Check sheet for the modelled part. Datum: model origin and axes. Units: mm. A direction names the side the tool comes from. Give positions to 0.01 mm unless a question says otherwise; leave off trailing zeros. Write each loop counter-clockwise with the first axis right and the second up, starting at its lowest first coordinate (ties: lowest second). Pieces come first, ordered by that corner, then holes. Notation, with made-up numbers: (-19, 36.25) - (-8, 36.25) arc R17 cw to (-8, 56.25) - close; hole circle Ø9 at (-36.75, 8.5). An arc over 180 degrees is marked (long way). Return JSON: item names as keys, results as strings. Group by question number.
```python
from build123d import *

# Parameters (mm, degrees)
F0_W     = 43.2
F0_H     = 4
F1_DEPTH = 1
F0_W_2   = 15.8
F0_H_2   = 2
F0_H_3   = 8.5
F2_DEPTH = 2.5
F3_DEPTH = 5
F4_DEPTH = 8


with BuildPart() as f1:
    # F0 (on Top) → F1 (new body)
    with BuildSketch(Plane.XY):
        Polygon((59, 16.5), (59, 24.5), (43.2, 24.5), (43.2, 20.5), (43.2, 16.5), align=None)
        with Locations((21.6, 22.5)):
            Rectangle(F0_W, F0_H)
    extrude(amount=F1_DEPTH)



with BuildPart() as f1b:
    # F0 (on Top) → F1, piece 2 (new body)
    with BuildSketch(Plane.XY):
        Polygon((59, 0), (59, 8), (43.2, 8), (43.2, 4), (43.2, 0), align=None)
        with Locations((21.6, 2)):
            Rectangle(F0_W, F0_H)
    extrude(amount=F1_DEPTH)


with BuildPart() as f1_1:
    add(f1.part)

    add(f1b.part)  # F2 merges F1b
    # F0 (on Top) → F2 (join)
    with BuildSketch(Plane.XY):
        with Locations((51.1, 25.5)):
            Rectangle(F0_W_2, F0_H_2)
        with Locations((51.1, 12.25)):
            Rectangle(F0_W_2, F0_H_3)
        with Locations((51.1, -1)):
            Rectangle(F0_W_2, F0_H_2)
        Polygon((61, 26.5), (59, 26.5), (59, 24.5), (59, 16.5), (59, 8), (59, 0), (59, -2), (61, -2), align=None)
    extrude(amount=F2_DEPTH)

    # F0 (on Top) → F3 (join)
    with BuildSketch(Plane.XY):
        Polygon((43.2, 8), (43.2, 16.5), (43.2, 20.5), (0, 20.5), (0, 4), (43.2, 4), align=None)
    extrude(amount=F3_DEPTH)

    # F0 (on Top) → F4 (join)
    with BuildSketch(Plane.XY):
        Polygon((43.2, 24.5), (43.2, 26.5), (-2, 26.5), (-2, -2), (43.2, -2), (43.2, 0), (0, 0), (0, 4), (0, 20.5), (0, 24.5), align=None)
    extrude(amount=F4_DEPTH)


solid = f1_1.part
```
Item 1: Mould release check, pull along Y, two halves, no side actions. Record for faces 1 (the face through (36, 2, 1)), 2 (the face through (23, 26.5, 4)), 3 (the face through (43.2, -1, 5)): +Y half, -Y half, draft (parallel to the pull), parting line (faces both ways), or undercut.
Item 2: Depth check by flat-ended pin: pin 1 (3 mm diameter, centred on x = 34.5, y = 23.5, fed in from +Z); pin 2 (9 mm diameter, centred on x = 54, y = 7.5, fed in from +Z); pin 3 (4 mm diameter, centred on x = 35.5, y = 4, fed in from +Z); pin 4 (2 mm diameter, centred on y = 25, z = 6.5, fed in from +X). Enter the tip coordinate at first touch or a pass-through.
Item 3: Section check C-C on z = 6.5. Record the cut outline in (x, y), plus the area to 3 significant figures.
Item 4: Material ranges on line 1 along Y through (x, z) = (10, 2.25); line 2 along Y through (x, z) = (27.5, 6.25); line 3 along Z through (x, y) = (27, 17.5), recorded low to high. Write a range as from..to.
Item 5: Section check B-B on y = 18.5. Record the cut outline in (x, z), plus the area to 3 significant figures.
Item 6: Access from +Z, -Z, +X, -X, +Y, -Y to the whole of each face (thin tool, end or side, straight path). Record for faces 4 (the face through (43.2, 25, 5)), 5 (the face through (22, 20.5, 3)), 6 (the face through (61, 12, 1)).
Item 7: Section check D-D on x = 53.5. Record the cut outline in (y, z), plus the area to 4 significant figures.
Item 8: Section check A-A on x = 5. Record the cut outline in (y, z).
Reply:
{
 "1": {"face 1": "undercut", "face 2": "+Y half", "face 3": "draft"},
 "2": {"pin 1": "z = 8", "pin 2": "z = 2.5", "pin 3": "z = 5", "pin 4": "x = 43.2"},
 "3": {"outline": "(-2, -2) - (43.2, -2) - (43.2, 0) - (0, 0) - (0, 24.5) - (43.2, 24.5) - (43.2, 26.5) - (-2, 26.5) - close", "area": "230 mm²"},
 "4": {"line 1": "-2..0, 4..20.5, 24.5..26.5", "line 2": "-2..0, 24.5..26.5", "line 3": "0..5"},
 "5": {"outline": "(-2, 0) - (61, 0) - (61, 2.5) - (59, 2.5) - (59, 1) - (43.2, 1) - (43.2, 5) - (0, 5) - (0, 8) - (-2, 8) - close", "area": "253 mm²"},
 "6": {"face 4": "+Z, +X, +Y, -Y", "face 5": "+Z", "face 6": "+Z, -Z, +X, +Y, -Y"},
 "7": {"outline": "(-2, 0) - (26.5, 0) - (26.5, 2.5) - (24.5, 2.5) - (24.5, 1) - (16.5, 1) - (16.5, 2.5) - (8, 2.5) - (8, 1) - (0, 1) - (0, 2.5) - (-2, 2.5) - close", "area": "47.25 mm²"},
 "8": {"outline": "(-2, 0) - (26.5, 0) - (26.5, 8) - (24.5, 8) - (24.5, 1) - (20.5, 1) - (20.5, 5) - (4, 5) - (4, 1) - (0, 1) - (0, 8) - (-2, 8) - close"}
}
